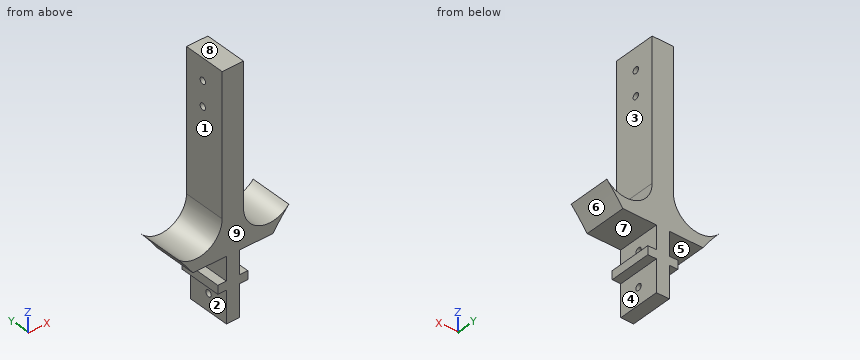
```python
from build123d import *

# Parameters (mm, degrees)
BOSS_EXTRU_1_DEPTH      = 20
ESQUISSE3_R             = 1.5
ENL_V_MAT_EXTRU_3_DEPTH = 20
ESQUISSE4_R             = 1.5
ENL_V_MAT_EXTRU_4_DEPTH = 10
ESQUISSE5_R             = 1.5
ENL_V_MAT_EXTRU_5_DEPTH = 10


with BuildPart() as part:
    # Esquisse1 → Boss.-Extru.1 (new body)
    with BuildSketch(Plane(origin=(0, 0, 0), x_dir=(1, 0, 0), z_dir=(0, 1, 0))):
        with BuildLine():
            Line((-3, 84.398281038), (-3, 69.398281038))
            Line((-3, 69.398281038), (-7, 69.398281038))
            Line((-7, 69.398281038), (-7, 65.398281038))
            Line((-7, 65.398281038), (-3, 65.398281038))
            Line((-3, 65.398281038), (-3, 54.398281038))
            Line((-3, 54.398281038), (-18.71, 54.398281038))
            ThreePointArc((-18.71, 54.398281038), (-22.308577777, 49.499317693), (-26.183329952, 44.81574006))
            ThreePointArc((-26.183329952, 44.81574006), (-12.83252844, 48.159570073), (-5, 36.842476876))
            Line((-5, 36.842476876), (-5, -28.467834127))
            Line((-5, -28.467834127), (0, -28.467834127))
            Line((0, -28.467834127), (0, 84.398281038))
            Line((0, 84.398281038), (-3, 84.398281038))
        make_face()
    boss_extru_1 = extrude(amount=BOSS_EXTRU_1_DEPTH)

    # Symétrie1: Boss.-Extru.1 across plane
    add(boss_extru_1.mirror(Plane(origin=(0, 20, -84.398281038), x_dir=(0, 0, 1), z_dir=(-1, 0, 0))))

    # Esquisse3 → Enlèv. mat.-Extru.3 (cut)
    with BuildSketch(Plane.ZY.offset(3)):
        with Locations((-76.398281038, 10)):
            Circle(ESQUISSE3_R)
        with Locations((-60.398281038, 10)):
            Circle(ESQUISSE3_R)
    extrude(amount=-ENL_V_MAT_EXTRU_3_DEPTH, mode=Mode.SUBTRACT)

    # Esquisse4 → Enlèv. mat.-Extru.4 (cut)
    with BuildSketch(Plane(origin=(5, 0, 0), x_dir=(0, 0, -1), z_dir=(1, 0, 0))):
        with Locations((-18.354301853, 10.844529297)):
            Circle(ESQUISSE4_R)
    extrude(amount=-ENL_V_MAT_EXTRU_4_DEPTH, mode=Mode.SUBTRACT)

    # Esquisse5 → Enlèv. mat.-Extru.5 (cut)
    with BuildSketch(Plane(origin=(5, 0, 0), x_dir=(0, 0, -1), z_dir=(1, 0, 0))):
        with Locations((-6.902461617, 10.844529297)):
            Circle(ESQUISSE5_R)
    extrude(amount=-ENL_V_MAT_EXTRU_5_DEPTH, mode=Mode.SUBTRACT)


solid = part.part
```
Source: CAD feature listing. Evaluate the final solid. Frame: model axes, mm. Face numbers are marked on the shaded views. A direction names the side the tool comes from. Give positions to 0.01 mm unless a question says otherwise; leave off trailing zeros. Write each loop counter-clockwise with the first axis right and the second up, starting at its lowest first coordinate (ties: lowest second). Pieces come first, ordered by that corner, then holes. Notation, with made-up numbers: (79, 56.25) - (126, 56.25) arc R18 cw to (126, 76.25) - close; hole circle Ø7 at (76.5, -17). An arc over 180 degrees is marked (long way). One line per item, written item: value. Start each with the question number.
Q1. First-contact query: pin 1 Ø1 at (x, y) = (-14, 12.5) entering from +Z; pin 2 Ø5.5 at (y, z) = (14.5, -61.5) entering from -X; pin 3 Ø1 at (x, y) = (18, 7.5) entering from -Z; pin 4 Ø10 at (x, z) = (13, -10.5) entering from +Y. Flat tips, straight axial feed; report the tip coordinate or a pass-through.
Q2. Section query B-B, the plane z = -46.5. Return the cut outline in (x, y).
Q3. Draft query along Z for the marked faces 6, 7, 8 and 9. Return one class per face: +Z half, -Z half, draft (parallel to the pull), parting line (faces both ways), or undercut.
Q4. Material intervals for probe 1 along X at (y, z) = (6, -46.5); probe 2 along Z at (x, y) = (-8, 2.25); probe 3 along Z at (x, y) = (17.5, 9.25), sorted ascending. Write a range as from..to.
Q5. Section query D-D, the plane z = 1. Return the cut outline in (x, y).
Q6. Set-up query: the marked faces 1, 2, 3, 4 and 5. Return all of +Z, -Z, +X, -X, +Y, -Y with unobstructed straight access to the full face (end or side cutting, diameter ignored); none if empty.
Q7. Section query C-C, the plane x = 21. Return the cut outline in (y, z).
Q8. Section query A-A, the plane y = 14.75. Return the cut outline in (x, z), then the cut area to 3 significant figures.
Answer:
1. pin 1: stops at z = -48.39
1. pin 2: stops at x = -3
1. pin 3: stops at z = -54.4
1. pin 4: passes through
2. outline: (-24.74, 0) - (-24.37, 0) - (-24.37, 20) - (-24.74, 20) - close; (-9.82, 0) - (9.82, 0) - (9.82, 20) - (-9.82, 20) - close; (24.37, 0) - (24.74, 0) - (24.74, 20) - (24.37, 20) - close
3. face 6: -Z half
3. face 7: undercut
3. face 8: +Z half
3. face 9: draft
4. probe 1: x = -24.74..-24.37, -9.82..9.82, 24.37..24.74
4. probe 2: z = -54.4..-44.81
4. probe 3: z = -54.4..-48.93
5. outline: (-5, 0) - (5, 0) - (5, 20) - (-5, 20) - close
6. face 1: +Z, -X, +Y, -Y
6. face 2: -Z, -X, +Y, -Y
6. face 3: +Z, +X, +Y, -Y
6. face 4: -Z, +X, +Y, -Y
6. face 5: -X, +Y, -Y
7. outline: (0, -51.21) - (20, -51.21) - (20, -48.29) - (0, -48.29) - close
8. outline: (-26.18, -44.82) arc R105.5 cw to (-18.71, -54.4) - (-3, -54.4) - (-3, -65.4) - (-7, -65.4) - (-7, -69.4) - (-3, -69.4) - (-3, -84.4) - (3, -84.4) - (3, -69.4) - (7, -69.4) - (7, -65.4) - (3, -65.4) - (3, -54.4) - (18.71, -54.4) arc R105.5 cw to (26.18, -44.82) arc R12.09 cw to (5, -36.84) - (5, 28.47) - (-5, 28.47) - (-5, -36.84) arc R12.09 cw to start
8. area: 1,280 mm2
